```python
from build123d import *

# Parameters (mm, degrees)
SKETCH_1_W          = 10
SKETCH_1_H          = 15
SKETCH_1_W_2        = 8
SKETCH_1_H_2        = 13
EXTRUDE_1_DEPTH     = 40
SKETCH_2_R          = 1.5
SKETCH_2_R_2        = 4
CUT_EXTRUDE_1_DEPTH = 11
SKETCH_3_R          = 1.5
CUT_EXTRUDE_2_DEPTH = 16


with BuildPart() as part:
    # 草图1 → 拉伸-薄壁1 (new body)
    with BuildSketch(Plane.XY):
        with Locations((88.100313923, 48.436702161)):
            Rectangle(SKETCH_1_W, SKETCH_1_H)
        with Locations((88.100313923, 48.436702161)):
            Rectangle(SKETCH_1_W_2, SKETCH_1_H_2, mode=Mode.SUBTRACT)
    extrude(amount=EXTRUDE_1_DEPTH)

    # 草图2 → 切除-拉伸1 (cut, through all)
    with BuildSketch(Plane.ZY.offset(-83.100313923)):
        with Locations((5, 48.436702161)):
            Circle(SKETCH_2_R)
        with Locations((27, 48.436702161)):
            Circle(SKETCH_2_R)
        with Locations((15, 48.436702161)):
            Circle(SKETCH_2_R_2)
    extrude(amount=-CUT_EXTRUDE_1_DEPTH, mode=Mode.SUBTRACT)

    # 草图3 → 切除-拉伸2 (cut, through all)
    with BuildSketch(Plane.XZ.offset(-40.936702161)):
        with Locations((88.100313923, 35)):
            Circle(SKETCH_3_R)
    extrude(amount=-CUT_EXTRUDE_2_DEPTH, mode=Mode.SUBTRACT)


solid = part.part
```
Model file for the job. Use its own axes, mm. A direction names the side the tool comes from. Give positions to 0.01 mm unless a question says otherwise; leave off trailing zeros. Write each loop counter-clockwise with the first axis right and the second up, starting at its lowest first coordinate (ties: lowest second). Pieces come first, ordered by that corner, then holes. Notation, with made-up numbers: M -2,31.5 L 8,31.5 A23 cw 8,64.5 Z; hole C 20.25,-10.75 d2. An arc over 180 degrees is marked long. Use a Markdown table: item, result.
1) Pin check, flat tips, straight feed: pin 1 (6.5 mm diameter, centred on y = 48.44, z = 15, fed in from +X); pin 2 (3.5 mm diameter, centred on y = 48.44, z = 5, fed in from +X). Stop position of each tip, or through.
Responses:
| item | result |
|---|---|
| pin 1 | passes through |
| pin 2 | stops at x = 93.1 |
2) Tool access for faces 1 (the cylindrical face through (92.59, 46, 11.83)), 2 (the flat face through (88, 54.937, 20)): list every direction of +Z, -Z, +X, -X, +Y, -Y with a clear straight run to the whole face (end or side of a thin tool).
Responses:
| item | result |
|---|---|
| face 1 | +X, -X |
| face 2 | +Z, -Z |
3) Cut at B-B (z = 35). List the corners of the cut face in (x, y), and give its area (3 significant figures).
Responses:
| item | result |
|---|---|
| outline | M 83.1,40.94 L 86.6,40.94 L 86.6,41.94 L 84.1,41.94 L 84.1,54.94 L 86.6,54.94 L 86.6,55.94 L 83.1,55.94 Z; M 89.6,40.94 L 93.1,40.94 L 93.1,55.94 L 89.6,55.94 L 89.6,54.94 L 92.1,54.94 L 92.1,41.94 L 89.6,41.94 Z |
| area | 40.0 mm2 |
4) Cut at C-C (y = 42.75). List the corners of the cut face in (x, z), and give its area (3 significant figures).
Responses:
| item | result |
|---|---|
| outline | M 83.1,0 L 84.1,0 L 84.1,40 L 83.1,40 Z; M 92.1,0 L 93.1,0 L 93.1,40 L 92.1,40 Z |
| area | 80.0 mm2 |
5) Cut at D-D (z = 22). List the corners of the cut face in (x, y), and give its area (3 significant figures).
Responses:
| item | result |
|---|---|
| outline | M 83.1,40.94 L 93.1,40.94 L 93.1,55.94 L 83.1,55.94 Z; hole M 84.1,41.94 L 92.1,41.94 L 92.1,54.94 L 84.1,54.94 Z |
| area | 46.0 mm2 |
6) Pull direction X, two halves, no side cores. Call faces 3 (the flat face through (88, 55.937, 20)), 4 (the cylindrical face through (86.6, 41.43, 35.07)), 5 (the flat face through (83.1, 48, 20)): +X half, -X half, draft (parallel to the pull), parting line (faces both ways), or undercut.
Responses:
| item | result |
|---|---|
| face 3 | draft |
| face 4 | undercut |
| face 5 | -X half |
7) Drill centre lines: line 1 (X direction, y = 45.5, z = 3); line 2 (Y direction, x = 92.8, z = 15); line 3 (Y direction, x = 90.5, z = 35.5). Where is each one in solid material? Low to high. Write a range as from..to.
Responses:
| item | result |
|---|---|
| line 1 | x = 83.1..84.1, 92.1..93.1 |
| line 2 | y = 40.94..44.44, 52.44..55.94 |
| line 3 | y = 40.94..41.94, 54.94..55.94 |
8) Cut at A-A (x = 86). List the corners of the cut face in (y, z), and give its area (3 significant figures).
Responses:
| item | result |
|---|---|
| outline | M 40.94,0 L 41.94,0 L 41.94,40 L 40.94,40 Z; M 54.94,0 L 55.94,0 L 55.94,40 L 54.94,40 Z |
| area | 80.0 mm2 |
